from build123d import *

# Parameters (mm, degrees)
F0_W     = 33.12
F0_H     = 22.44
F1_DEPTH = 13.28
F0_W_2   = 17.88
F0_R     = 4.5
F2_DEPTH = 3
F3_T     = -3
F4_W     = 8
F4_H     = 16.44
F5_DEPTH = 3
F6_R     = 5


# Not quite as in the source:
# - a shell that OpenCascade refuses in one call is made with other operations: the cavity is built on its own and cut out
# - a feature names something its author has since deleted; it is built from what else it names


with BuildPart() as f1:
    # F0 (on Top) → F1 (new body)
    with BuildSketch(Plane.XY):
        Polygon((30.6844967631, 22.44), (30.6844967631, 0), (53.1244967631, 0), (53.1244967631, 32.44), (30.6844967631, 32.44), align=None)
        with Locations((14.1244967631, 11.22)):
            Rectangle(F0_W, F0_H)
    extrude(amount=F1_DEPTH)

    # F0 (on Top) → F2 (join)
    with BuildSketch(Plane.XY):
        with Locations((-11.3755032369, 11.22)):
            Rectangle(F0_W_2, F0_H)
        with Locations((-10.8755032369, 11.22)):
            Circle(F0_R, mode=Mode.SUBTRACT)
    extrude(amount=F2_DEPTH)

    # F3: a shell. OpenCascade refuses it in one call, so the cavity is built on its own and cut out:
    # the body offset inwards by the wall thickness, plus a prism from it out through each open face.
    f3_core = offset(f1.part, amount=F3_T, kind=Kind.INTERSECTION, mode=Mode.PRIVATE)
    f3_exits = [f3_core.faces().sort_by_distance(p)[0] for p in [
        (0.564497, 11.22, 6.64),
        (41.904497, 29.44, 6.64),
    ]]
    add(f3_core, mode=Mode.SUBTRACT)
    extrude(f3_exits, amount=-F3_T, mode=Mode.SUBTRACT)

    # F4 (on face) → F5 (cut)
    with BuildSketch(Plane.XY.offset(13.28)):
        with Locations((29.6844967631, 11.22)):
            Rectangle(F4_W, F4_H)
        Polygon((50.1244967631, 27.44), (33.6844967631, 27.44), (33.6844967631, 19.44), (33.6844967631, 3), (50.1244967631, 3), align=None)
    extrude(amount=-F5_DEPTH, mode=Mode.SUBTRACT)

    # F6
    f6_edges = [f1.edges().sort_by_distance(p)[0] for p in [
        (53.124497, 0, 6.64),
        (30.684497, 22.44, 6.64),
        (33.684497, 19.44, 8.14),
        (50.124497, 3, 8.14),
        (-20.315503, 22.44, 1.5),
        (-20.315503, 0, 1.5),
    ]]
    fillet(f6_edges, radius=F6_R)


solid = f1.part
Build history of the part. All positions in model axes, mm. A direction names the side the tool comes from. Round coordinates to 2 decimals unless told otherwise and drop trailing zeros. Write each loop counter-clockwise with the first axis right and the second up, starting at its lowest first coordinate (ties: lowest second). Pieces come first, ordered by that corner, then holes. Notation, with made-up numbers: M 62,-35 L 78,-35 A18 cw 78,-10 Z; hole C -17,7 d9. An arc over 180 degrees is marked long. Answer in a Markdown table with one row per item.
1. Which spindle directions (+Z, -Z, +X, -X, +Y, -Y) get a long thin tool onto all of the face, cutting with end or side? Do faces 1 (the face through (12, 11, 10.28)), 2 (the face through (9, 22.44, 7)), 3 (the face through (-2.436, 11, 11)), 4 (the face through (50.124, 20, 8)). Say none if no direction does.
Geometry check:
| item | result |
|---|---|
| face 1 | -X |
| face 2 | +Z, -Z, -X, +Y |
| face 3 | +Z, -X, +Y, -Y |
| face 4 | none |
2. Saw through at D-D (x = 7). List the corners of the cut face in (y, z), and give its area (3 significant figures).
Geometry check:
| item | result |
|---|---|
| outline | M 0,0 L 22.44,0 L 22.44,13.28 L 0,13.28 Z; hole M 3,3 L 19.44,3 L 19.44,10.28 L 3,10.28 Z |
| area | 178 mm2 |
3. Probe L1, parallel to Y at x = 16.5, z = 8.5; L2, parallel to Y at x = 22, z = 11.75; L3, parallel to X at y = 16, z = 7. List the from-to ranges inside material, lowest first. Write a range as [from, to].
Geometry check:
| item | result |
|---|---|
| L1 | [0, 3], [19.44, 22.44] |
| L2 | [0, 22.44] |
| L3 | [50.12, 53.12] |
4. Saw through at A-A (z = 7.5). List the corners of the cut face in (x, y).
Geometry check:
| item | result |
|---|---|
| outline | M -2.44,0 L 48.12,0 A5 ccw 53.12,5 L 53.12,32.44 L 50.12,32.44 L 50.12,8 A5 cw 45.12,3 L -2.44,3 Z; M -2.44,19.44 L 28.68,19.44 A5 ccw 33.68,24.44 L 33.68,32.44 L 30.68,32.44 L 30.68,27.44 A5 cw 25.68,22.44 L -2.44,22.44 Z |
5. Saw through at C-C (y = 29). List the corners of the cut face in (x, z).
Geometry check:
| item | result |
|---|---|
| outline | M 30.68,0 L 53.12,0 L 53.12,13.28 L 30.68,13.28 Z; hole M 33.68,3 L 50.12,3 L 50.12,10.28 L 33.68,10.28 Z |
6. Mould opens along Z. For faces 5 (the face through (33.684, 28, 7)), 6 (the face through (13, 19.44, 7)), 7 (the face through (24, 13, 0)), 8 (the face through (-6.583, 12.572, 1.479)) say: +Z half, -Z half, draft (parallel to the pull), parting line (faces both ways), or undercut.
Geometry check:
| item | result |
|---|---|
| face 5 | undercut |
| face 6 | undercut |
| face 7 | -Z half |
| face 8 | draft |
7. Saw through at B-B (y = 11.22). List the corners of the cut face in (x, z), and give its area (3 significant figures).
Geometry check:
| item | result |
|---|---|
| outline | M -20.32,0 L -15.38,0 L -15.38,3 L -20.32,3 Z; M -6.38,0 L 53.12,0 L 53.12,13.28 L 50.12,13.28 L 50.12,3 L -6.38,3 Z; M -2.44,10.28 L 25.68,10.28 L 25.68,13.28 L -2.44,13.28 Z |
| area | 309 mm2 |
8. Flat gauge pins, fed straight in: P1, Ø4, axis at y = 29, z = 7.5, coming from the -X side; P2, Ø10.5, axis at x = -10.88, y = 11.22, coming from the +Z side; P3, Ø4, axis at y = 17, z = 9, coming from the -X side. Where does each tip first touch, or does it go through?
Geometry check:
| item | result |
|---|---|
| P1 | x = 30.67 |
| P2 | z = 3 |
| P3 | x = -2.44 |
